```python
from build123d import *

# Parameters (mm, degrees)
SKETCH1_W           = 5
SKETCH1_H           = 3
BOSS_EXTRUDE1_DEPTH = 2
CUT_EXTRUDE1_REACH  = 53.173
SKETCH2_R           = 1.5


with BuildPart() as part:
    # Sketch1 → Boss-Extrude1 (new body)
    with BuildSketch(Plane.XY):
        Polygon((33.4, -27.6), (33.4, -32.6), (25.4, -32.6), (25.4, -27.6), (10, -27.6), (10, -32.6), (-10, -32.6), (-10, -27.6), (-25.4, -27.6), (-25.4, -32.6), (-33.4, -32.6), (-33.4, -27.6), (-35, -27.6), (-35, -32.6), (-36.6, -32.6), (-39.394660298, -20.2), (-39.394660298, -18.6), (-33.4, -18.6), (-33.4, -16.6), (-25.4, -16.6), (-25.4, -18.6), (-10, -18.6), (-10, -16.6), (10, -16.6), (10, -18.6), (25.4, -18.6), (25.4, -16.6), (33.4, -16.6), (33.4, -18.6), (39.394660298, -18.6), (39.394660298, -20.2), (36.6, -32.6), (35, -32.6), (35, -27.6), align=None)
        with Locations((31.1, -23.1)):
            Rectangle(SKETCH1_W, SKETCH1_H, mode=Mode.SUBTRACT)
        with Locations((-31.1, -23.1)):
            Rectangle(SKETCH1_W, SKETCH1_H, mode=Mode.SUBTRACT)
    extrude(amount=BOSS_EXTRUDE1_DEPTH)

    # Sketch2 → Cut-Extrude1 (cut, up to next)
    with BuildSketch(Plane.XY.offset(2), mode=Mode.PRIVATE) as cut_extrude1_sk1:
        with Locations((12, -23.1)):
            Circle(SKETCH2_R)
    cut_extrude1_tool1 = extrude(cut_extrude1_sk1.sketch, amount=-CUT_EXTRUDE1_REACH, mode=Mode.PRIVATE) & part.part
    # Sketch2 → Cut-Extrude1 (cut, up to next)
    with BuildSketch(Plane.XY.offset(2), mode=Mode.PRIVATE) as cut_extrude1_sk2:
        with Locations((-12, -23.1)):
            Circle(SKETCH2_R)
    cut_extrude1_tool2 = extrude(cut_extrude1_sk2.sketch, amount=-CUT_EXTRUDE1_REACH, mode=Mode.PRIVATE) & part.part
    add(cut_extrude1_tool1.solids().sort_by_distance((12, -23.1, 2))[0], mode=Mode.SUBTRACT)
    add(cut_extrude1_tool2.solids().sort_by_distance((-12, -23.1, 2))[0], mode=Mode.SUBTRACT)


solid = part.part
```
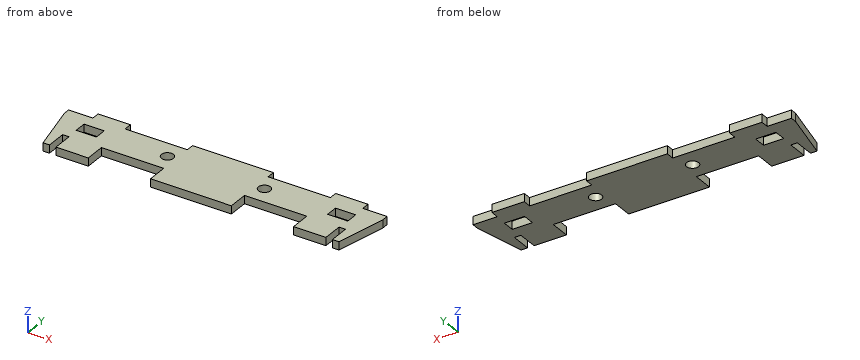
Model file for the job. Use its own axes, mm. Coordinates: 2 decimals unless noted, no trailing zeros. Write each loop counter-clockwise with the first axis right and the second up, starting at its lowest first coordinate (ties: lowest second). Pieces come first, ordered by that corner, then holes. Notation, with made-up numbers: (0, -31.75) - (58, -31.75) arc R28 cw to (58, 7.25) - close; hole circle Ø3 at (24, 76.5). An arc over 180 degrees is marked (long way). Use a Markdown table: item, result. Add a question column.
Item 1: Drill centre lines: line 1 along X through (y, z) = (-18.25, 1.5); line 2 along Y through (x, z) = (-12, 1.55); line 3 along X through (y, z) = (-23, 1.6). Where is each one in solid material? Low to high.
Item 2: Drop flat-ended pins along their axis: pin 1 (0.6 mm diameter, centred on y = -30, z = 1, fed in from +X); pin 2 (0.6 mm diameter, centred on y = -18, z = 0.5, fed in from -X); pin 3 (1 mm diameter, centred on y = -31, z = 1, fed in from +X). Give the stop position or say it passes through.
Item 3: Band-saw the part on B-B, the plane y = -23.1. Write the cut outline in (x, z).
Item 4: Band-saw the part on D-D, the plane z = 1.1. Give the number of separate pieces and of enclosed holes in the cut face, and give its area (3 significant figures).
Item 5: Band-saw the part on A-A, the plane x = 29.5. Write the cut outline in (y, z).
Item 6: Band-saw the part on C-C, the plane x = 12. Write the cut outline in (y, z), and give its area (3 significant figures).
A:
| question | item | result |
|---|---|---|
| 1 | line 1 | x = -33.4 to -25.4, -10 to 10, 25.4 to 33.4 |
| 1 | line 2 | y = -27.6 to -24.6, -21.6 to -18.6 |
| 1 | line 3 | x = -38.76 to -33.6, -28.6 to -13.5, -10.5 to 10.5, 13.5 to 28.6, 33.6 to 38.76 |
| 2 | pin 1 | stops at x = 37.25 |
| 2 | pin 2 | stops at x = -33.4 |
| 2 | pin 3 | stops at x = 37.07 |
| 3 | outline | (-38.74, 0) - (-33.6, 0) - (-33.6, 2) - (-38.74, 2) - close; (-28.6, 0) - (-13.5, 0) - (-13.5, 2) - (-28.6, 2) - close; (-10.5, 0) - (10.5, 0) - (10.5, 2) - (-10.5, 2) - close; (13.5, 0) - (28.6, 0) - (28.6, 2) - (13.5, 2) - close; (33.6, 0) - (38.74, 0) - (38.74, 2) - (33.6, 2) - close |
| 4 | separate pieces | 1 |
| 4 | enclosed holes | 4 |
| 4 | area | 926 mm² |
| 5 | outline | (-32.6, 0) - (-24.6, 0) - (-24.6, 2) - (-32.6, 2) - close; (-21.6, 0) - (-16.6, 0) - (-16.6, 2) - (-21.6, 2) - close |
| 6 | outline | (-27.6, 0) - (-24.6, 0) - (-24.6, 2) - (-27.6, 2) - close; (-21.6, 0) - (-18.6, 0) - (-18.6, 2) - (-21.6, 2) - close |
| 6 | area | 12.0 mm² |
